```python
from build123d import *

# Parameters (mm, degrees)
F0_R     = 8.5
F1_DEPTH = 15
F2_R     = 8.5
F3_DEPTH = 4
F4_SIZE  = 1


with BuildPart() as f1:
    # F0 (on Top) → F1 (new body)
    with BuildSketch(Plane.XY):
        with BuildLine():
            Line((10, -11.1803398875), (10, 11.1803398875))
            ThreePointArc((10, 11.1803398875), (0, 15), (-10, 11.1803398875))
            Line((-10, 11.1803398875), (-10, -11.1803398875))
            ThreePointArc((-10, -11.1803398875), (0, -15), (10, -11.1803398875))
        make_face()
        Circle(F0_R, mode=Mode.SUBTRACT)
    extrude(amount=F1_DEPTH)

    # F2 (on face) → F3 (cut)
    with BuildSketch(Plane.XY.offset(15)):
        with BuildLine():
            Line((10, -7.5), (10, 7.5))
            ThreePointArc((10, 7.5), (0, 12.5), (-10, 7.5))
            Line((-10, 7.5), (-10, -7.5))
            ThreePointArc((-10, -7.5), (0, -12.5), (10, -7.5))
        make_face()
        Circle(F2_R, mode=Mode.SUBTRACT)
    extrude(amount=-F3_DEPTH, mode=Mode.SUBTRACT)

    # F4
    f4_edges = [f1.edges().sort_by_distance(p)[0] for p in [
        (0, -15, 15),
        (0, 15, 15),
    ]]
    chamfer(f4_edges, length=F4_SIZE)


solid = f1.part
```
For this review, take the finished solid that the model builds, in its own axes (mm). A direction names the side the tool comes from. Coordinates: 2 decimals unless noted, no trailing zeros. Write each loop counter-clockwise with the first axis right and the second up, starting at its lowest first coordinate (ties: lowest second). Pieces come first, ordered by that corner, then holes.
(1) Add section C-C on z = 9. Give the boundary of the cut face in (x, y).
(2) Add section D-D on y = 0. Give the boundary of the cut face in (x, z).
(3) For pin 1 Ø10 at (x, y) = (-3.5, 6) entering from +Z; pin 2 Ø1 at (x, z) = (-2, 2.5) entering from +Y; pin 3 Ø2 at (x, z) = (7, 5.5) entering from +Y, all flat-tipped, find the tip position at first contact; note any pin that passes through.
(4) Tool access review of faces 4 (the face through (-0.2, -14.2, 14.8)), 5 (the face through (0.2, 12.5, 13)): name each direction out of +Z, -Z, +X, -X, +Y, -Y from which nothing blocks a thin tool from reaching the whole face with its end or side.
(5) Wall thickness on probe 1 along Y at (x, z) = (0, 4.75); probe 2 along Z at (x, y) = (8.5, 8.5); probe 3 along Y at (x, z) = (6.25, 10.75): over which ranges is each line inside the solid? List them lowest first.
(6) Add section B-B on x = 0. Give the boundary of the cut face in (y, z), then the cut area to 3 significant figures.
(7) The part is to be moulded in two halves that separate along X. For faces 1 (the face through (-9, 0, 0)), 2 (the face through (0.2, 14.2, 14.8)), 3 (the face through (4.57, 7.167, 5.423)), say which applies: +X half, -X half, draft (parallel to the pull), parting line (faces both ways), or undercut.
(8) Add section A-A on y = 3.5. Give the boundary of the cut face in (x, z), then the cut area to 3 significant figures.
Answer sheet:
1. outline: (-10, -11.18) arc R15 ccw to (10, -11.18) - (10, 11.18) arc R15 ccw to (-10, 11.18) - close; hole circle Ø17 at (0, 0)
2. outline: (-10, 0) - (-8.5, 0) - (-8.5, 11) - (-10, 11) - close; (8.5, 0) - (10, 0) - (10, 11) - (8.5, 11) - close
3. pin 1: stops at z = 11
3. pin 2: stops at y = 14.92
3. pin 3: stops at y = 13.75
4. face 4: +Z, -Y
4. face 5: +Z
5. probe 1: y = -15 to -8.5, 8.5 to 15
5. probe 2: z = 0 to 11
5. probe 3: y = -13.64 to -5.76, 5.76 to 13.64
6. outline: (-15, 0) - (-8.5, 0) - (-8.5, 11) - (-12.5, 11) - (-12.5, 15) - (-14, 15) - (-15, 14) - close; (8.5, 0) - (15, 0) - (15, 14) - (14, 15) - (12.5, 15) - (12.5, 11) - (8.5, 11) - close
6. area: 162 mm2
7. face 1: draft
7. face 2: parting line
7. face 3: undercut
8. outline: (-10, 0) - (-7.75, 0) - (-7.75, 11) - (-10, 11) - close; (7.75, 0) - (10, 0) - (10, 11) - (7.75, 11) - close
8. area: 49.6 mm2
